For this review, take the finished solid that the model builds, in its own axes (mm). A direction names the side the tool comes from. Coordinates: 2 decimals unless noted, no trailing zeros. Write each loop counter-clockwise with the first axis right and the second up, starting at its lowest first coordinate (ties: lowest second). Pieces come first, ordered by that corner, then holes. Notation, with made-up numbers: M -29.75,0.5 L -21.75,0.5 A22 ccw -21.75,9.5 Z; hole C -29.5,-12 d6. An arc over 180 degrees is marked long. One line per question, with ' | ' between items.
Autodesk Inventor part; units mm, degrees
ref_plane "YZ Plane" through (0, 0, 0) normal (1, 0, 0) x (0, 1, 0)
ref_plane "XZ Plane" through (0, 0, 0) normal (0, 1, 0) x (-1, 0, 0)
ref_plane "XY Plane" through (0, 0, 0) normal (0, 0, 1) x (1, 0, 0)
sketch "Skizze1" plane through (0, 0, 0) normal (0, 1, 0) x (-1, 0, 0)
  line L0 (3.5, -2.0207) -> (0, -4.0415)
  line L1 (0, -4.0415) -> (-3.5, -2.0207)
  line L2 (-3.5, -2.0207) -> (-3.5, 2.0207)
  line L3 (-3.5, 2.0207) -> (0, 4.0415)
  line L4 (0, 4.0415) -> (3.5, 2.0207)
  line L5 (3.5, 2.0207) -> (3.5, -2.0207)
  point P0 (0, 0)
  point P1 (0, 0)
  dimension "d0" = 7
extrude "Extrusion1" add sketch "Skizze1" along normal blind 38
sketch "Skizze2" plane through (0, 38, 0) normal (0, 1, 0) x (1, 0, 0)
  point P0 (0, 0)
  point P1 (0, 0)
hole "Bohrung1" at (0, 38, 0) direction (0, -1, 0) diameter 3.242 depth 11.8 tip angle 118
sketch "Skizze3" plane through (0, 0, 0) normal (0, -1, 0) x (1, 0, 0)
  point P0 (0, 0)
  point P1 (0, 0)
hole "Bohrung2" at (0, 0, 0) direction (0, 1, 0) diameter 3.242 depth 11.8 tip angle 118
chamfer "Fasen1" distance 0.5 angle 45 12 edges at (-1.75, 38, 3.0311) (1.75, 38, 3.0311) (3.5, 38, 0) (1.75, 38, -3.0311) (-1.75, 38, -3.0311) (-3.5, 38, 0) (-3.5, 0, 0) (-1.75, 0, 3.0311) (1.75, 0, 3.0311) (3.5, 0, 0) (1.75, 0, -3.0311) (-1.75, 0, -3.0311)
properties part number "Abstandsbolzen 38mm" material "Aluminium 6061"
1. Take a section at C-C on z = -2.75. State the section outline as (x, y) points.
Computed values:
outline: M -2.24,0.5 L -1.24,0 L 1.24,0 L 2.24,0.5 L 2.24,37.5 L 1.24,38 L -1.24,38 L -2.24,37.5 Z
2. Take a section at B-B on y = 24. State the section outline as (x, z) points, plus the area to 3 significant figures.
Computed values:
outline: M -3.5,-2.02 L 0,-4.04 L 3.5,-2.02 L 3.5,2.02 L 0,4.04 L -3.5,2.02 Z | area: 42.4 mm2
3. Take a section at A-A on y = 8.5. State the section outline as (x, z) points.
Computed values:
outline: M -3.5,-2.02 L 0,-4.04 L 3.5,-2.02 L 3.5,2.02 L 0,4.04 L -3.5,2.02 Z; hole C 0,0 d3.24
4. Machinability: for faces 4 (the flat face through (1.65, 37.75, -2.8)), 5 (the cylindrical face through (1.438, 5.983, -0.748)), which of the approach directions +Z, -Z, +X, -X, +Y, -Y give a long, thin tool a straight path to every point of the face, cutting with its end or side? Answer none if there is none.
Computed values:
face 4: -Z, +X, +Y | face 5: -Y
5. Clearance check with flat-ended pins moving along their axes: P1, Ø3, axis at x = 0, z = 0, coming from the +Y side; P2, Ø1, axis at x = -1.5, y = 12, coming from the +Z side. State where each tip first meets the part, or that it passes through.
Computed values:
P1: stops at y = 26.13 | P2: stops at z = 3.46
6. Draft analysis for pull direction Z (two halves, no side actions). For faces 1 (the flat face through (1.726, 18.741, -3.045)), 2 (the flat face through (1.4, 38, -1.5)), 3 (the conical face through (-0.25, 25.395, 0.13)), state which applies: pulls with the +Z half, pulls with the -Z half, needs draft (parallel to the pull), parting line crosses it, or undercut.
Computed values:
face 1: pulls with the -Z half | face 2: needs draft | face 3: undercut
7. For line 1 along X through (y, z) = (31.25, 0); line 2 along Z through (x, y) = (-0.25, 35.5); line 3 along X through (y, z) = (33, -1), list the stretches that pass through material, from the lowest coordinate up.
Computed values:
line 1: x = -3.5 to -1.62, 1.62 to 3.5 | line 2: z = -3.9 to -1.6, 1.6 to 3.9 | line 3: x = -3.5 to -1.28, 1.28 to 3.5
